The listing builds one solid part. Answer for the finished solid, in the listing's coordinates (mm). A direction names the side the tool comes from. Coordinates: 2 decimals unless noted, no trailing zeros. Loops run counter-clockwise (first coordinate to the right, second up) from the corner with the lowest first, then second, coordinate; pieces in that order, holes last. Notation, with made-up numbers: (58, 20.5) -> (110, 20.5) arc R19 cw to (110, 55.5) -> close; hole circle Ø9 at (55, 28). An arc over 180 degrees is marked (long way). Answer in a Markdown table with one row per item.
```python
from build123d import *

# Parameters (mm, degrees)
F0_R     = 15.375
F1_DEPTH = 6
F0_R_2   = 17.25
F2_DEPTH = 2
F3_T     = -2.4
F4_R     = 1


with BuildPart() as f1:
    # F0 (on Top) → F1 (new body)
    with BuildSketch(Plane.XY):
        Circle(F0_R)
    extrude(amount=F1_DEPTH)

    # F0 (on Top) → F2 (join)
    with BuildSketch(Plane.XY):
        Circle(F0_R_2)
        Circle(F0_R, mode=Mode.SUBTRACT)
    extrude(amount=F2_DEPTH)

    # F3
    f3_openings = [f1.faces().sort_by_distance(p)[0] for p in [
        (0, 0, 6),
    ]]
    offset(amount=F3_T, openings=f3_openings)

    # F4
    f4_edges = [f1.edges().sort_by_distance(p)[0] for p in [
        (-15.375, 0, 6),
        (-12.975, 0, 2.4),
    ]]
    fillet(f4_edges, radius=F4_R)


solid = f1.part
```
Item 1: Find the intervals of material crossed by probe 1 along Y at (x, z) = (0, 4.2) (3 decimals); probe 2 along Z at (x, y) = (-2, 3); probe 3 along Y at (x, z) = (10.5, 4.75), in increasing order.
Findings below:
| item | result |
|---|---|
| probe 1 | y = -15.375 to -12.975, 12.975 to 15.375 |
| probe 2 | z = 0 to 2.4 |
| probe 3 | y = -11.23 to -7.62, 7.62 to 11.23 |
Item 2: Determine the mould class of faces 1 (the face through (11.986, -4.97, 4.682)), 2 (the face through (-2, 13, 6)), 3 (the face through (16.453, 5.181, 0.986)) for opening direction X: +X half, -X half, draft (parallel to the pull), parting line (faces both ways), or undercut.
Findings below:
| item | result |
|---|---|
| face 1 | undercut |
| face 2 | draft |
| face 3 | parting line |
Item 3: A cutting plane is placed at B-B, the plane z = 4.5. Determine the outline of the cut face in (x, y) (3 decimals), plus the area to 3 significant figures.
Findings below:
| item | result |
|---|---|
| outline | circle Ø30.75 at (0, 0); hole circle Ø25.95 at (0, 0) |
| area | 214 mm2 |
Item 4: A tool of negligible diameter and unlimited length cuts with its end or side. For faces 4 (the face through (0, 0, 2.4)), 5 (the face through (0, 0, 0)), from which of +Z, -Z, +X, -X, +Y, -Y can it reach the whole face along a straight path? Write none if from no direction.
Findings below:
| item | result |
|---|---|
| face 4 | +Z |
| face 5 | -Z, +X, -X, +Y, -Y |
Item 5: A cutting plane is placed at A-A, the plane y = 0. Determine the outline of the cut face in (x, z) (3 decimals).
Findings below:
| item | result |
|---|---|
| outline | (-17.25, 0) -> (17.25, 0) -> (17.25, 2) -> (15.375, 2) -> (15.375, 5) arc R1 ccw to (14.375, 6) -> (12.975, 6) -> (12.975, 3.4) arc R1 cw to (11.975, 2.4) -> (-11.975, 2.4) arc R1 cw to (-12.975, 3.4) -> (-12.975, 6) -> (-14.375, 6) arc R1 ccw to (-15.375, 5) -> (-15.375, 2) -> (-17.25, 2) -> close |
Item 6: Flat-ended cylindrical pins translate along their axes: pin 1 Ø8 at (x, y) = (6.5, 3) entering from -Z; pin 2 Ø1 at (x, z) = (-9.5, 1.5) entering from +Y. Find the tip coordinate at first contact, or state that the pin passes through.
Findings below:
| item | result |
|---|---|
| pin 1 | stops at z = 0 |
| pin 2 | stops at y = 14.72 |
